Source: CAD feature listing. Evaluate the final solid. Frame: model axes, mm. Face numbers are marked on the shaded views. Give positions to 0.01 mm unless a question says otherwise; leave off trailing zeros. Order: outer loops, then holes, each group sorted by start corner. A loop starts at its lowest first (then second) coordinate and runs counter-clockwise, first axis right, second up.
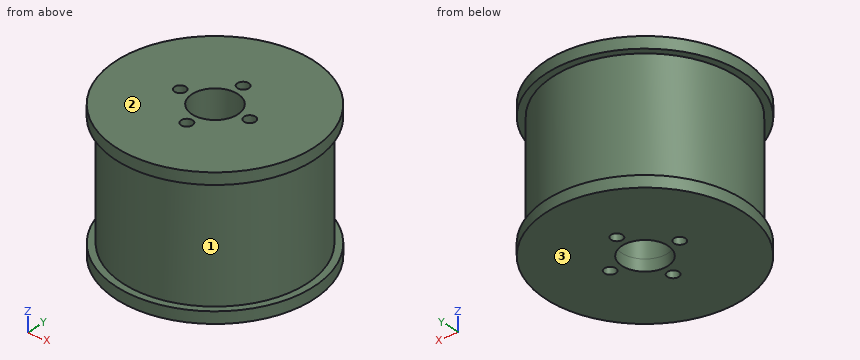
from build123d import *

# Parameters (mm, degrees)
SKETCH1_R           = 40
SKETCH1_R_2         = 10
BOSS_EXTRUDE1_DEPTH = 50
SKETCH2_R           = 43
SKETCH2_R_2         = 10
BOSS_EXTRUDE2_DEPTH = 5
SKETCH3_R           = 43
SKETCH3_R_2         = 10
BOSS_EXTRUDE3_DEPTH = 5
SKETCH4_R           = 2.5
CUT_EXTRUDE1_DEPTH  = 61


with BuildPart() as part:
    # Sketch1 → Boss-Extrude1 (new body)
    with BuildSketch(Plane.XY):
        Circle(SKETCH1_R)
        Circle(SKETCH1_R_2, mode=Mode.SUBTRACT)
    extrude(amount=BOSS_EXTRUDE1_DEPTH)

    # Sketch2 → Boss-Extrude2 (add)
    with BuildSketch(Plane.XY.offset(50)):
        Circle(SKETCH2_R)
        Circle(SKETCH2_R_2, mode=Mode.SUBTRACT)
    extrude(amount=BOSS_EXTRUDE2_DEPTH)

    # Sketch3 → Boss-Extrude3 (add)
    with BuildSketch(Plane(origin=(0, 0, 0), x_dir=(-1, 0, 0), z_dir=(0, 0, -1))):
        Circle(SKETCH3_R)
        Circle(SKETCH3_R_2, mode=Mode.SUBTRACT)
    extrude(amount=BOSS_EXTRUDE3_DEPTH)

    # Sketch4 → Cut-Extrude1 (cut, through all)
    with BuildSketch(Plane.XY.offset(55)):
        with Locations((0, 15)):
            Circle(SKETCH4_R)
        with Locations((15, 0)):
            Circle(SKETCH4_R)
        with Locations((0, -15)):
            Circle(SKETCH4_R)
        with Locations((-15, 0)):
            Circle(SKETCH4_R)
    extrude(amount=-CUT_EXTRUDE1_DEPTH, mode=Mode.SUBTRACT)


solid = part.part
1) Ray query, L1, parallel to Y at x = 0, z = 8; L2, parallel to Y at x = -4, z = 44; L3, parallel to Y at x = 17, z = 46. Return the intervals inside material, ascending.
Checks:
L1: y = -40 to -17.5, -12.5 to -10, 10 to 12.5, 17.5 to 40
L2: y = -39.8 to -9.17, 9.17 to 39.8
L3: y = -36.21 to -1.5, 1.5 to 36.21
2) Section query C-C on y = -15. Output: boundary loops of the cut face in (x, z), and give its area (3 significant figures).
Checks:
outline: (-40.3, -5) - (-2.5, -5) - (-2.5, 55) - (-40.3, 55) - (-40.3, 50) - (-37.08, 50) - (-37.08, 0) - (-40.3, 0) - close; (2.5, -5) - (40.3, -5) - (40.3, 0) - (37.08, 0) - (37.08, 50) - (40.3, 50) - (40.3, 55) - (2.5, 55) - close
area: 4,210 mm2
3) Section query A-A on x = 0. Output: boundary loops of the cut face in (y, z), and give its area (3 significant figures).
Checks:
outline: (-43, -5) - (-17.5, -5) - (-17.5, 55) - (-43, 55) - (-43, 50) - (-40, 50) - (-40, 0) - (-43, 0) - close; (-12.5, -5) - (-10, -5) - (-10, 55) - (-12.5, 55) - close; (10, -5) - (12.5, -5) - (12.5, 55) - (10, 55) - close; (17.5, -5) - (43, -5) - (43, 0) - (40, 0) - (40, 50) - (43, 50) - (43, 55) - (17.5, 55) - close
area: 3,060 mm2
4) First-contact query: pin 1 Ø3 at (x, y) = (0, 15) entering from +Z; pin 2 Ø1.5 at (y, z) = (31, 33.5) entering from +X; pin 3 Ø2 at (y, z) = (30.5, 43) entering from +X; pin 4 Ø1 at (y, z) = (-1, 8) entering from +X. Flat tips, straight axial feed; report the tip coordinate or a pass-through.
Checks:
pin 1: passes through
pin 2: stops at x = 26.17
pin 3: stops at x = 27.01
pin 4: stops at x = 40
5) Pull-direction query (Z, two-part tool) for the marked faces 1, 2 and 3; classes: +Z half, -Z half, draft (parallel to the pull), parting line (faces both ways), or undercut.
Checks:
face 1: undercut
face 2: +Z half
face 3: -Z half
